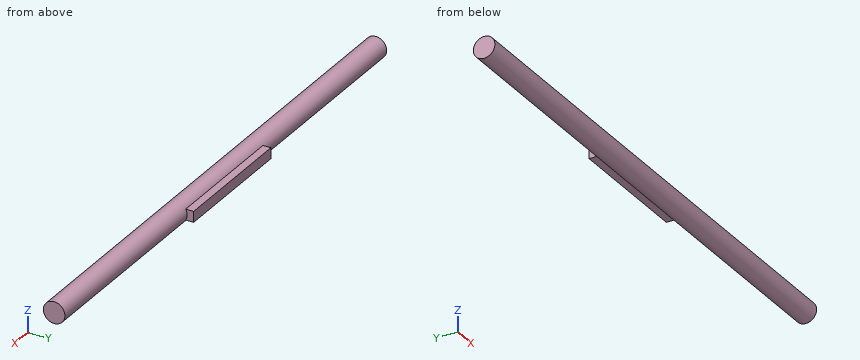
from build123d import *

# Parameters (mm, degrees)
SKETCH2_R                       = 5
SHAFT_DEPTH                     = 125
SHAFT_DEPTH_BACK                = 125
SKETCH3_W                       = 5
SKETCH3_H                       = 8
SHAFT_KEY_FOR_BICEPS_DEPTH      = 30
SHAFT_KEY_FOR_BICEPS_DEPTH_BACK = 30


with BuildPart() as part:
    # Sketch2 → Shaft (new body, two sides)
    with BuildSketch(Plane(origin=(0, 0, 0), x_dir=(0, 0, -1), z_dir=(1, 0, 0))) as shaft_sk:
        Circle(SKETCH2_R)
    extrude(amount=SHAFT_DEPTH)
    extrude(shaft_sk.sketch, amount=-SHAFT_DEPTH_BACK)

    # Sketch3 → Shaft Key for Biceps (add, two sides)
    with BuildSketch(Plane(origin=(0, 0, 0), x_dir=(0, 0, -1), z_dir=(1, 0, 0))) as shaft_key_for_biceps_sk:
        with Locations((0, 4)):
            Rectangle(SKETCH3_W, SKETCH3_H)
    extrude(amount=SHAFT_KEY_FOR_BICEPS_DEPTH)
    extrude(shaft_key_for_biceps_sk.sketch, amount=-SHAFT_KEY_FOR_BICEPS_DEPTH_BACK)


solid = part.part
The model under review builds one solid part; all positions refer to its coordinate system, in mm. Round coordinates to 2 decimals unless told otherwise and drop trailing zeros. Order: outer loops, then holes, each group sorted by start corner. A loop starts at its lowest first (then second) coordinate and runs counter-clockwise, first axis right, second up. Notation, with made-up numbers: (2.25, 26) -> (57.25, 26) arc R26 cw to (57.25, 62) -> close; hole circle Ø6 at (-17.75, -14.5). An arc over 180 degrees is marked (long way). Return JSON: item names as keys, results as strings.
1. Take a section at C-C (y = -2.75). Write out the cut boundary in (x, z), then the cut area to 3 significant figures.
Answer block:
{"outline": "(-125, -4.18) -> (125, -4.18) -> (125, 4.18) -> (-125, 4.18) -> close", "area": "2,090 mm²"}
2. Take a section at D-D (x = 83.5). Write out the cut boundary in (y, z).
Answer block:
{"outline": "circle Ø10 at (0, 0)"}
3. For L1, parallel to Y at x = -105, z = 0; L2, parallel to X at y = 6.75, z = -1.5; L3, parallel to Z at x = -12, y = 7.5, list the stretches that pass through material, from the lowest coordinate up. Write a range as [from, to].
Answer block:
{"L1": "y = [-5, 5]", "L2": "x = [-30, 30]", "L3": "z = [-2.5, 2.5]"}
4. Take a section at B-B (x = -19.5). Write out the cut boundary in (y, z).
Answer block:
{"outline": "(4.33, -2.5) -> (8, -2.5) -> (8, 2.5) -> (4.33, 2.5) arc R5 ccw (long way) to start"}
5. Insertion check: P1, Ø4, axis at x = 60.5, z = 3.5, coming from the +Y side; P2, Ø1.1, axis at y = 6.5, z = 0, coming from the -X side; P3, Ø1, axis at x = 2, y = -2, coming from the -Z side. Each pin has a flat end and moves straight along its axis. Give the tip position at first contact, or say it passes through.
Answer block:
{"P1": "stops at y = 4.77", "P2": "stops at x = -30", "P3": "stops at z = -4.77"}
6. Take a section at A-A (z = 0). Write out the cut boundary in (x, y).
Answer block:
{"outline": "(-125, -5) -> (125, -5) -> (125, 5) -> (30, 5) -> (30, 8) -> (-30, 8) -> (-30, 5) -> (-125, 5) -> close"}
